The figure shows three views and two pictorial views of one solid part (mm, origin at its lowest corner). Answer the questions. Give positions to 0.01 mm unless a question says otherwise; leave off trailing zeros. Write each loop counter-clockwise with the first axis right and the second up, starting at its lowest first coordinate (ties: lowest second). Pieces come first, ordered by that corner, then holes. Notation, with made-up numbers: (7, 51) - (33, 51) arc R32 ccw to (33, 78) - close; hole circle Ø11 at (49.5, 12). An arc over 180 degrees is marked (long way). Write each question's results on one line, items separated by ' | '. Start each with the question number.
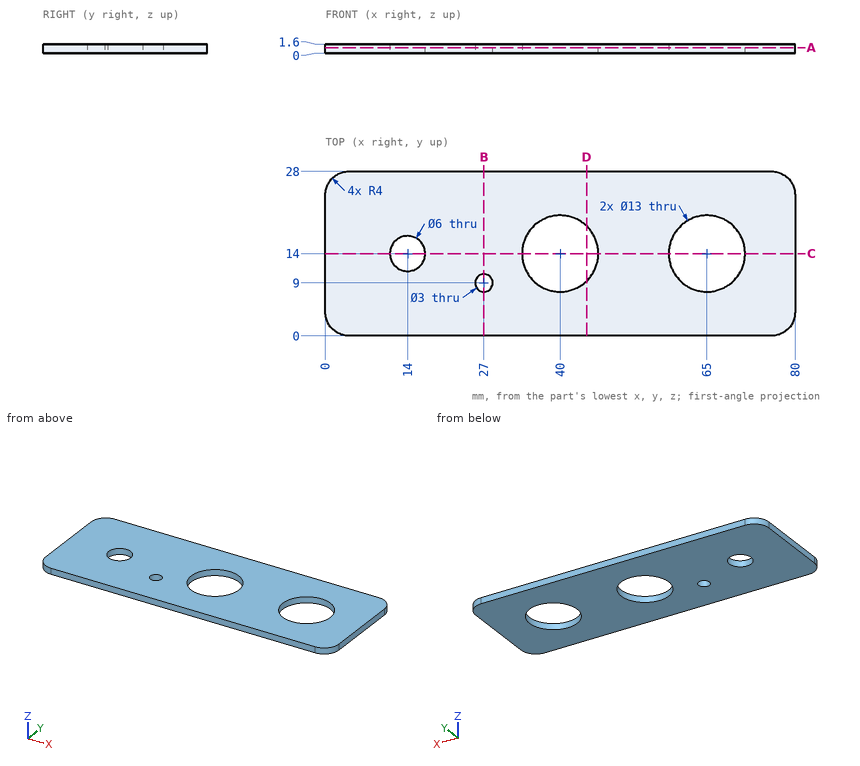
Q1. A cutting plane is placed at A-A, the plane z = 1. Write down the section's boundary in (x, y), and give its area (3 significant figures).
Q2. A cutting plane is placed at B-B, the plane x = 27. Write down the section's boundary in (y, z), and give its area (3 significant figures).
Q3. Given pin 1 (15 mm diameter, centred on x = 65, y = 14, fed in from +Z), flat-ended and moving along its own axis, determine where the tip first touches the part or whether it passes through.
Q4. A cutting plane is placed at C-C, the plane y = 14. Write down the section's boundary in (x, z).
Q5. A cutting plane is placed at D-D, the plane x = 44.5. Write down the section's boundary in (y, z).
Q6. Consider L1, parallel to Y at x = 65, z = 1; L2, parallel to Y at x = 14, z = 0.65; L3, parallel to X at y = 15.5, z = 1.1. Determine where each line is inside the solid, lowest interval first.
Result:
1) outline: (0, 4) arc R4 ccw to (4, 0) - (76, 0) arc R4 ccw to (80, 4) - (80, 24) arc R4 ccw to (76, 28) - (4, 28) arc R4 ccw to (0, 24) - close; hole circle Ø6 at (14, 14); hole circle Ø3 at (27, 9); hole circle Ø13 at (40, 14); hole circle Ø13 at (65, 14) | area: 1,930 mm2
2) outline: (0, 0) - (7.5, 0) - (7.5, 1.6) - (0, 1.6) - close; (10.5, 0) - (28, 0) - (28, 1.6) - (10.5, 1.6) - close | area: 40.0 mm2
3) pin 1: stops at z = 1.6
4) outline: (0, 0) - (11, 0) - (11, 1.6) - (0, 1.6) - close; (17, 0) - (33.5, 0) - (33.5, 1.6) - (17, 1.6) - close; (46.5, 0) - (58.5, 0) - (58.5, 1.6) - (46.5, 1.6) - close; (71.5, 0) - (80, 0) - (80, 1.6) - (71.5, 1.6) - close
5) outline: (0, 0) - (9.31, 0) - (9.31, 1.6) - (0, 1.6) - close; (18.69, 0) - (28, 0) - (28, 1.6) - (18.69, 1.6) - close
6) L1: y = 0 to 7.5, 20.5 to 28 | L2: y = 0 to 11, 17 to 28 | L3: x = 0 to 11.4, 16.6 to 33.68, 46.32 to 58.68, 71.32 to 80
